Design review of the part shown in the three views and the two pictorial views. Dimensions are in mm from the part's minimum x, y and z. A direction names the side the tool comes from. Coordinates: 2 decimals unless noted, no trailing zeros. Order: outer loops, then holes, each group sorted by start corner. A loop starts at its lowest first (then second) coordinate and runs counter-clockwise, first axis right, second up. Notation, with made-up numbers: (-24.75, 79.5) -> (32.25, 79.5) arc R18 ccw to (32.25, 103.5) -> close; hole circle Ø4 at (74.25, -3). An arc over 180 degrees is marked (long way). Answer as a JSON object with one key per item and string values. Group by question number.
1) Machinability: for the marked faces 1, 2, 3 and 4, which of the approach directions +Z, -Z, +X, -X, +Y, -Y give a long, thin tool a straight path to every point of the face, cutting with its end or side? Answer none if there is none.
2) Add section C-C, the plane x = 28. Write out the cut boundary in (y, z).
3) Add section A-A, the plane x = 20. Write out the cut boundary in (y, z).
4) Add section B-B, the plane y = 15. Count the separate pieces of the cut face and the enclosed holes in it, then the cut area to 3 significant figures.
5) Add section D-D, the plane z = 15. Write out the cut boundary in (x, y), then the cut area to 3 significant figures.
6) Draft analysis for pull direction Z (two halves, no side actions). For the marked faces 5, 6, 7 and 8, state which applies: +Z half, -Z half, draft (parallel to the pull), parting line (faces both ways), or undercut.
7) Wall thickness on L1, parallel to Z at x = 57, y = 15; L2, parallel to Z at x = 34, y = 14.75: over which ranges is each line inside the solid? List them lowest first.
8) For pin 1 (18 mm diameter, centred on x = 28.5, y = 10, fed in from -Z); pin 2 (1 mm diameter, centred on x = 29.5, z = 4, fed in from +Y); pin 3 (1.5 mm diameter, centred on y = 7.5, z = 25, fed in from -X); pin 4 (3 mm diameter, centred on x = 56, y = 18.5, fed in from +Z), all flat-tipped, find the tip position at first contact; note any pin that passes through.
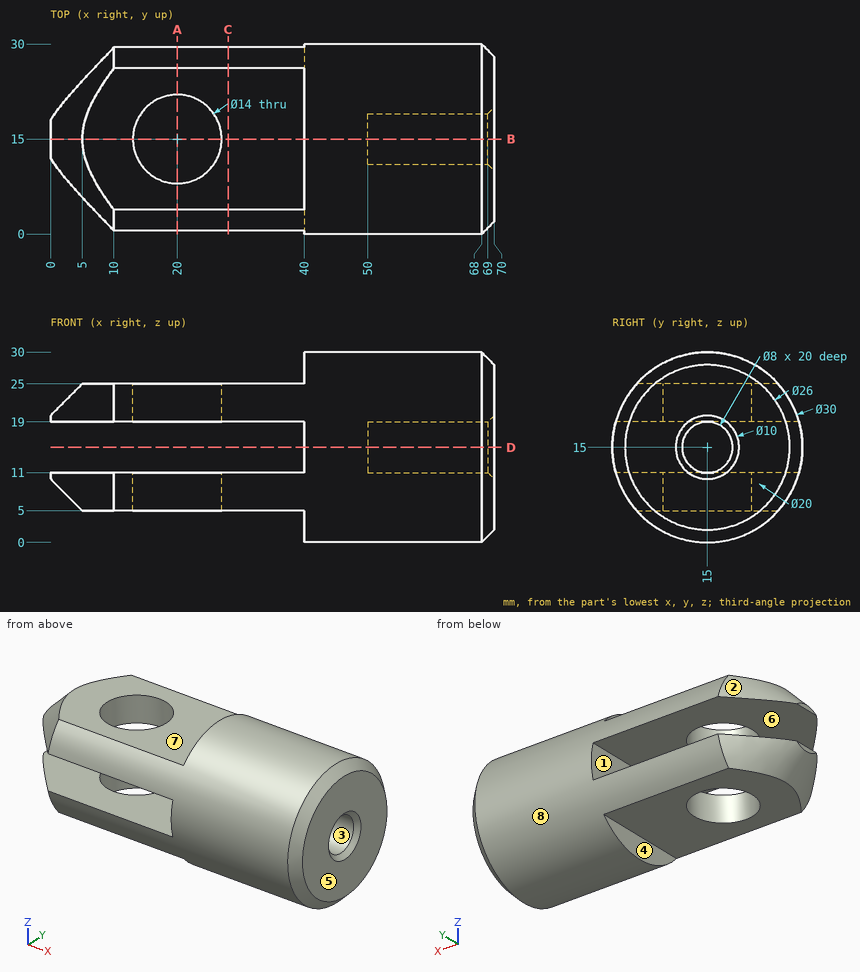
Output values:
{
 "1": {"face 1": "-X, +Y, -Y", "face 2": "+Z, -X", "face 3": "+X", "face 4": "-Z, -X, +Y, -Y"},
 "2": {"outline": "(0.54, 11) arc R15 ccw to (3.82, 5) -> (26.18, 5) arc R15 ccw to (29.46, 11) -> close; (0.54, 19) -> (29.46, 19) arc R15 ccw to (26.18, 25) -> (3.82, 25) arc R15 ccw to start"},
 "3": {"outline": "(0.54, 11) arc R15 ccw to (3.82, 5) -> (8, 5) -> (8, 11) -> close; (0.54, 19) -> (8, 19) -> (8, 25) -> (3.82, 25) arc R15 ccw to start; (22, 5) -> (26.18, 5) arc R15 ccw to (29.46, 11) -> (22, 11) -> close; (22, 19) -> (29.46, 19) arc R15 ccw to (26.18, 25) -> (22, 25) -> close"},
 "4": {"separate pieces": "3", "enclosed holes": "0", "area": "1,020 mm²"},
 "5": {"outline": "(40, 0) -> (68, 0) -> (70, 2) -> (70, 10) -> (69, 11) -> (50, 11) -> (50, 19) -> (69, 19) -> (70, 20) -> (70, 28) -> (68, 30) -> (40, 30) -> close", "area": "735 mm²"},
 "6": {"face 5": "draft", "face 6": "undercut", "face 7": "+Z half", "face 8": "parting line"},
 "7": {"L1": "z = 0 to 11, 19 to 30", "L2": "z = 5 to 11, 19 to 25"},
 "8": {"pin 1": "stops at z = 5", "pin 2": "passes through", "pin 3": "stops at x = 6.75", "pin 4": "stops at z = 29.87"}
}
